Source: CAD feature listing. Evaluate the final solid. Frame: model axes, mm. A direction names the side the tool comes from. Give positions to 0.01 mm unless a question says otherwise; leave off trailing zeros. Write each loop counter-clockwise with the first axis right and the second up, starting at its lowest first coordinate (ties: lowest second). Pieces come first, ordered by that corner, then holes. Notation, with made-up numbers: M 14,43 L 71,43 A3 ccw 71,48 Z; hole C 77.5,-27.75 d11. An arc over 180 degrees is marked long. Return JSON: item names as keys, results as strings.
```python
from build123d import *

# Parameters (mm, degrees)
F1_DEPTH = 63.5
F2_DEPTH = 7.9375
F3_R     = 6.35
F0_W     = 25.194674
F0_H     = 19.05
F4_DEPTH = 25.4


with BuildPart() as f1:
    # F0 (on Front) → F1 (new body, symmetric)
    with BuildSketch(Plane.XZ):
        Polygon((-41.275, -9.525), (41.275, -9.525), (41.275, 9.525), (22.225, 9.525), (-41.275, 9.525), align=None)
    extrude(amount=F1_DEPTH, both=True)

    # F0 (on Front) → F2 (join, symmetric)
    with BuildSketch(Plane.XZ):
        with BuildLine():
            add(Edge.make_bspline(
                [(-41.275, 9.525), (-40.449119, 34.956452), (0.491742, 58.062427), (51.965438, 61.538236)],
                knots=[0, 0, 0, 0, 108.503557, 108.503557, 108.503557, 108.503557], degree=3))
            Line((-41.275, 9.525), (22.225, 9.525))
            Line((22.225, 9.525), (22.225, 27.0002))
            ThreePointArc((22.225, 27.0002), (30.684679, 49.789285), (51.965438, 61.538236))
        make_face()
    extrude(amount=F2_DEPTH, both=True)

    # F3
    f3_edges = [f1.edges().sort_by_distance(p)[0] for p in [
        (41.275, -63.5, 0),
        (-41.275, -63.5, 0),
        (41.275, 63.5, 0),
        (-41.275, 63.5, 0),
    ]]
    fillet(f3_edges, radius=F3_R)

    # F0 (on Front) → F4 (join, symmetric)
    with BuildSketch(Plane.XZ):
        with BuildLine():
            Line((22.225, 9.525), (41.275, 9.525))
            Line((41.275, 9.525), (41.275, 27.0002))
            ThreePointArc((41.275, 27.0002), (45.92468, 38.22552), (57.15, 42.8752))
            Line((57.15, 42.8752), (60.325, 42.8752))
            Line((60.325, 42.8752), (60.325, 61.9252))
            add(Edge.make_bspline(
                [(51.965438, 61.538236), (54.723241, 61.724459), (57.511278, 61.854334), (60.325, 61.9252)],
                knots=[108.503557, 108.503557, 108.503557, 108.503557, 114.316845, 114.316845, 114.316845, 114.316845], degree=3))
            ThreePointArc((51.965438, 61.538236), (30.684679, 49.789285), (22.225, 27.0002))
            Line((22.225, 27.0002), (22.225, 9.525))
        make_face()
        with Locations((72.922337, 52.4002)):
            Rectangle(F0_W, F0_H)
    extrude(amount=F4_DEPTH, both=True)

    # F0 (on Front) → F5 (revolve)
    with BuildSketch(Plane.XZ):
        Polygon((85.519674, 66.675), (85.519674, 61.9252), (85.519674, 42.8752), (85.519674, 38.1), (111.125, 38.1), (111.125, 66.675), align=None)
    revolve(axis=Axis((85.519674, 0, 52.3875), (0, 0, 1)))


solid = f1.part
```
1) Draft query along X for faces 1 (the face through (86, 0, 38.1)), 2 (the face through (45.8, -0.4, 38.1)), 3 (the face through (22.225, 17, 18)). Return one class per face: released by +X, released by -X, zero draft, split by the parting line, or undercut.
Numbers:
{"face 1": "zero draft", "face 2": "undercut", "face 3": "released by -X"}
2) Set-up query: faces 4 (the face through (66, 20, 61.925)), 5 (the face through (22.225, -17, 18)), 6 (the face through (39.464, -61.59, 0.133)). Return all of +Z, -Z, +X, -X, +Y, -Y with unobstructed straight access to the full face (end or side cutting, diameter ignored); none if empty.
Numbers:
{"face 4": "+Z, -X, +Y", "face 5": "+Z, -X, -Y", "face 6": "+Z, -Z, +X, -Y"}
3) Line query: line 1 (X direction, y = 18.5, z = 28); line 2 (Z direction, x = -13.5, y = 44.5) (3 decimals); line 3 (Y direction, x = 19, z = 46.5). Output: solid intervals per line, ascending. Write a range as [from, to].
Numbers:
{"line 1": "x = [22.24, 41.31]", "line 2": "z = [-9.525, 9.525]", "line 3": "y = [-7.94, 7.94]"}
4) Cut plane A-A, the plane x = 79. Return the cut outline in (y, z) (3 decimals), then the cut area to 3 significant figures.
Numbers:
{"outline": "M -25.4,42.875 L -24.761,42.875 L -24.761,38.1 L 24.761,38.1 L 24.761,42.875 L 25.4,42.875 L 25.4,61.925 L 24.761,61.925 L 24.761,66.675 L -24.761,66.675 L -24.761,61.925 L -25.4,61.925 Z", "area": "1,440 mm²"}
5) Contact query for flat-ended pins moving along their axis: pin 1 Ø1.5 at (x, z) = (15, 54) entering from +Y; pin 2 Ø1.5 at (x, y) = (73.5, -11) entering from -Z; pin 3 Ø6 at (y, z) = (7.5, 26) entering from -X; pin 4 Ø15.5 at (x, z) = (55.5, 26) entering from +Y. Output: stop coordinate, or through.
Numbers:
{"pin 1": "stops at y = 7.94", "pin 2": "stops at z = 38.1", "pin 3": "stops at x = -37.06", "pin 4": "passes through"}
6) Cut plane B-B, the plane y = 40. Return the cut outline in (x, z) (3 decimals).
Numbers:
{"outline": "M -41.275,-9.525 L 41.275,-9.525 L 41.275,9.525 L -41.275,9.525 Z"}
